from build123d import *

# Parameters (mm, degrees)
SKETCH_1_W          = 64
SKETCH_1_H          = 64
EXTRUDE_1_DEPTH     = 5
FILLET_1_R          = 10
SKETCH_3_R          = 2.1
CUT_EXTRUDE_2_DEPTH = 10
SKETCH_2_R          = 10
CUT_EXTRUDE_3_DEPTH = 20


with BuildPart() as part:
    # 草图1 → 凸台-拉伸1 (new body)
    with BuildSketch(Plane(origin=(0, 0, 0), x_dir=(1, 0, 0), z_dir=(0, 1, 0))):
        Rectangle(SKETCH_1_W, SKETCH_1_H)
    extrude(amount=EXTRUDE_1_DEPTH)

    # 圆角1
    fillet_1_edges = [part.edges().sort_by_distance(p)[0] for p in [
        (32, 2.5, 32),
        (-32, 2.5, 32),
        (-32, 2.5, -32),
        (32, 2.5, -32),
    ]]
    fillet(fillet_1_edges, radius=FILLET_1_R)

    # 草图3 → 切除-拉伸2 (cut)
    with BuildSketch(Plane(origin=(0, 5, 0), x_dir=(1, 0, 0), z_dir=(0, 1, 0))):
        with Locations(Location((24.04163056, 24.04163056, 0), (0, 0, 270))):
            Circle(SKETCH_3_R)
        with Locations(Location((24.04163056, -24.04163056, 0), (0, 0, 270))):
            Circle(SKETCH_3_R)
        with Locations(Location((-24.04163056, -24.04163056, 0), (0, 0, 270))):
            Circle(SKETCH_3_R)
        with Locations(Location((-24.04163056, 24.04163056, 0), (0, 0, 270))):
            Circle(SKETCH_3_R)
    extrude(amount=-CUT_EXTRUDE_2_DEPTH, mode=Mode.SUBTRACT)

    # 草图2 → 切除-拉伸3 (cut)
    with BuildSketch(Plane(origin=(0, 5, 0), x_dir=(1, 0, 0), z_dir=(0, 1, 0))):
        with Locations(Location((0, 0, 0), (0, 0, 270))):
            Circle(SKETCH_2_R)
    extrude(amount=-CUT_EXTRUDE_3_DEPTH, mode=Mode.SUBTRACT)


solid = part.part
Read the model definition and answer for the solid it produces. Units are mm, in the model's axes. Coordinates: 2 decimals unless noted, no trailing zeros. Loops run counter-clockwise (first coordinate to the right, second up) from the corner with the lowest first, then second, coordinate; pieces in that order, holes last. Notation, with made-up numbers: (36, 54) -> (42, 54) arc R13 ccw to (42, 68) -> close; hole circle Ø2 at (76.5, 37.5). An arc over 180 degrees is marked (long way). Answer in a Markdown table with one row per item.
Item 1: A cutting plane is placed at B-B on x = 0. Determine the outline of the cut face in (y, z), plus the area to 3 significant figures.
Returned:
| item | result |
|---|---|
| outline | (0, -32) -> (5, -32) -> (5, -10) -> (0, -10) -> close; (0, 10) -> (5, 10) -> (5, 32) -> (0, 32) -> close |
| area | 220 mm^2 |
Item 2: Straight lines are drawn through the part: line 1 along Z through (x, y) = (23.5, 1.95); line 2 along Z through (x, y) = (-22.5, 3.8); line 3 along X through (y, z) = (2.95, 24). For each, find the intervals that lie inside material, in ascending order. Write a range as [from, to].
Returned:
| item | result |
|---|---|
| line 1 | z = [-31.89, -26.07], [-22.01, 22.01], [26.07, 31.89] |
| line 2 | z = [-31.99, -25.47], [-22.62, 22.62], [25.47, 31.99] |
| line 3 | x = [-31.8, -26.14], [-21.94, 21.94], [26.14, 31.8] |
Item 3: A cutting plane is placed at C-C on y = 2. Determine the outline of the cut face in (x, z).
Returned:
| item | result |
|---|---|
| outline | (-32, -22) arc R10 ccw to (-22, -32) -> (22, -32) arc R10 ccw to (32, -22) -> (32, 22) arc R10 ccw to (22, 32) -> (-22, 32) arc R10 ccw to (-32, 22) -> close; hole circle Ø4.2 at (-24.04, -24.04); hole circle Ø4.2 at (-24.04, 24.04); hole circle Ø20 at (0, 0); hole circle Ø4.2 at (24.04, -24.04); hole circle Ø4.2 at (24.04, 24.04) |
Item 4: For a pull along X with two mould halves and no side action, classify faces 1 (the cylindrical face through (-22.271, 2.535, -22.913)), 2 (the cylindrical face through (28.99, 2.54, 29.15)), 3 (the cylindrical face through (-29.15, 2.54, -28.99)), 4 (the flat face through (0, 2, 32)) as released by +X, released by -X, zero draft, split by the parting line, or undercut.
Returned:
| item | result |
|---|---|
| face 1 | undercut |
| face 2 | released by +X |
| face 3 | released by -X |
| face 4 | zero draft |
Item 5: This flat-tipped pin is pushed along its axis until it touches: P1, Ø4, axis at x = 24.04, z = 24.04, coming from the -Y side. Where does it stop, or does it pass through?
Returned:
| item | result |
|---|---|
| P1 | passes through |
Item 6: A cutting plane is placed at A-A on z = 0. Determine the outline of the cut face in (x, y).
Returned:
| item | result |
|---|---|
| outline | (-32, 0) -> (-10, 0) -> (-10, 5) -> (-32, 5) -> close; (10, 0) -> (32, 0) -> (32, 5) -> (10, 5) -> close |
